Read the model definition and answer for the solid it produces. Units are mm, in the model's axes. Face numbers are marked on the shaded views. A direction names the side the tool comes from. Coordinates: 2 decimals unless noted, no trailing zeros. Write each loop counter-clockwise with the first axis right and the second up, starting at its lowest first coordinate (ties: lowest second). Pieces come first, ordered by that corner, then holes. Notation, with made-up numbers: M 32.5,7 L 74.5,7 A20 ccw 74.5,22 Z; hole C 5,73.5 d7. An arc over 180 degrees is marked long. Write item = value, one per line.
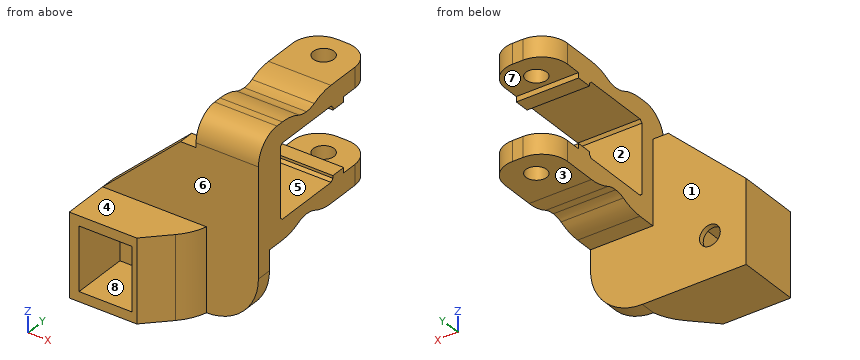
from build123d import *

# Parameters (mm, degrees)
ESQUISSE1_W                   = 30
ESQUISSE1_H                   = 40
BOSS_EXTRU_1_DEPTH            = 3
ESQUISSE8_W                   = 17
ESQUISSE8_H                   = 3.5
BOSS_EXTRU_2_DEPTH            = 20
ESQUISSE11_W                  = 3.5
ESQUISSE11_H                  = 20
ENL_V_MAT_EXTRU_9_DEPTH       = 5
ESQUISSE19_W                  = 12
ESQUISSE19_H                  = 20
BOSS_EXTRU_6_DEPTH            = 16.5
ESQUISSE20_W                  = 14.2
ESQUISSE20_H                  = 14.2
ENL_V_MAT_EXTRU_11_DEPTH      = 50.527769988
ESQUISSE29_W                  = 12
ESQUISSE29_H                  = 3
BOSS_EXTRU_9_DEPTH            = 17
ESQUISSE30_W                  = 12
ESQUISSE30_H                  = 23
BOSS_EXTRU_10_DEPTH           = 1
ESQUISSE31_W                  = 12
ESQUISSE31_H                  = 20
BOSS_EXTRU_11_DEPTH           = 1
ESQUISSE32_W                  = 12.2
ESQUISSE32_H                  = 2.9
ENL_V_MAT_EXTRU_12_DEPTH      = 50.527769988
ESQUISSE33_W                  = 12
ESQUISSE33_H                  = 3.9
BOSS_EXTRU_12_DEPTH           = 8
CONG_6_R                      = 5
ENL_V_MAT_EXTRU_14_DEPTH      = 53.417083332
ENL_V_MAT_EXTRU_14_DEPTH_BACK = 53.417083332
ESQUISSE36_R                  = 2
CHANFREIN1_SIZE               = 0.5
CONG_7_R                      = 5
ENL_V_MAT_EXTRU_15_DEPTH      = 54.712196008
CONG_8_R                      = 10
CONG_9_R                      = 10
ESQUISSE39_W                  = 30
ESQUISSE39_H                  = 3
BOSS_EXTRU_13_DEPTH           = 2
ESQUISSE40_W                  = 18
ESQUISSE40_H                  = 3
BOSS_EXTRU_14_DEPTH           = 2
ESQUISSE38_R                  = 2
ENL_V_MAT_EXTRU_16_DEPTH      = 61.207973065
ESQUISSE41_W                  = 14
ESQUISSE41_H                  = 16
ESQUISSE41_W_2                = 10
ESQUISSE41_H_2                = 12
BOSS_EXTRU_15_DEPTH           = 9
ESQUISSE42_W                  = 10
ESQUISSE42_H                  = 12
ENL_V_MAT_EXTRU_17_DEPTH      = 2
ESQUISSE43_W                  = 30
ESQUISSE43_H                  = 14
ENL_V_MAT_EXTRU_19_DEPTH      = 3
CONG_10_R                     = 10
ESQUISSE44_W                  = 6
ESQUISSE44_H                  = 16
BOSS_EXTRU_16_DEPTH           = 9
CHANFREIN2_SIZE               = 7
CONG_11_R                     = 10
ESQUISSE46_W                  = 10.2
ESQUISSE46_H                  = 12.2
ENL_V_MAT_EXTRU_20_DEPTH      = 11


with BuildPart() as part:
    # Esquisse1 → Boss.-Extru.1 (new body)
    with BuildSketch(Plane(origin=(0, 0, 0), x_dir=(1, 0, 0), z_dir=(0, 1, 0))):
        with Locations((15, 20)):
            Rectangle(ESQUISSE1_W, ESQUISSE1_H)
    extrude(amount=BOSS_EXTRU_1_DEPTH)

    # Esquisse8 → Boss.-Extru.2 (add)
    with BuildSketch(Plane(origin=(0, 3, 0), x_dir=(1, 0, 0), z_dir=(0, 1, 0))):
        with Locations((21.5, 11.375)):
            Rectangle(ESQUISSE8_W, ESQUISSE8_H)
    extrude(amount=BOSS_EXTRU_2_DEPTH)

    # Esquisse11 → Enlèv. mat.-Extru.9 (cut)
    with BuildSketch(Plane.ZY.offset(-13)):
        with Locations((-11.375, 13)):
            Rectangle(ESQUISSE11_W, ESQUISSE11_H)
    extrude(amount=-ENL_V_MAT_EXTRU_9_DEPTH, mode=Mode.SUBTRACT)

    # Esquisse19 → Boss.-Extru.6 (add)
    with BuildSketch(Plane.XY.offset(-9.625)):
        with Locations((24, 13)):
            Rectangle(ESQUISSE19_W, ESQUISSE19_H)
    extrude(amount=BOSS_EXTRU_6_DEPTH)

    # Esquisse20 → Enlèv. mat.-Extru.11 (cut, through all)
    with BuildSketch(Plane.ZY.offset(-18)):
        with Locations((-3.125, 13)):
            Rectangle(ESQUISSE20_W, ESQUISSE20_H)
    extrude(amount=-ENL_V_MAT_EXTRU_11_DEPTH, mode=Mode.SUBTRACT)

    # Esquisse29 → Boss.-Extru.9 (add)
    with BuildSketch(Plane.XY.offset(6.875)):
        with Locations((24, 1.5)):
            Rectangle(ESQUISSE29_W, ESQUISSE29_H)
    extrude(amount=-BOSS_EXTRU_9_DEPTH)

    # Esquisse30 → Boss.-Extru.10 (add)
    with BuildSketch(Plane.XY.offset(6.875)):
        with Locations((24, 11.5)):
            Rectangle(ESQUISSE30_W, ESQUISSE30_H)
    extrude(amount=BOSS_EXTRU_10_DEPTH)

    # Esquisse31 → Boss.-Extru.11 (add)
    with BuildSketch(Plane(origin=(0, 0, -13.125), x_dir=(-1, 0, 0), z_dir=(0, 0, -1))):
        with Locations((-24, 13)):
            Rectangle(ESQUISSE31_W, ESQUISSE31_H)
    extrude(amount=BOSS_EXTRU_11_DEPTH)

    # Esquisse32 → Enlèv. mat.-Extru.12 (cut, through all)
    with BuildSketch(Plane.ZY.offset(-18)):
        with Locations((-3.125, 21.55)):
            Rectangle(ESQUISSE32_W, ESQUISSE32_H)
    extrude(amount=-ENL_V_MAT_EXTRU_12_DEPTH, mode=Mode.SUBTRACT)

    # Esquisse33 → Boss.-Extru.12 (add)
    with BuildSketch(Plane(origin=(0, 23, 0), x_dir=(1, 0, 0), z_dir=(0, 1, 0))):
        with Locations((24, 12.175)):
            Rectangle(ESQUISSE33_W, ESQUISSE33_H)
        with Locations((24, -5.925)):
            Rectangle(ESQUISSE33_W, ESQUISSE33_H)
    extrude(amount=BOSS_EXTRU_12_DEPTH)

    # Congé6
    cong_6_edges = [part.edges().sort_by_distance(p)[0] for p in [
        (18, 31, -12.175),
        (30, 31, -12.175),
        (18, 31, 5.925),
        (30, 31, 5.925),
    ]]
    fillet(cong_6_edges, radius=CONG_6_R)

    # Esquisse36 → Enlèv. mat.-Extru.14 (cut, two sides: drawn at the far end of the back side and taken through both)
    with BuildSketch(Plane.XY.offset(-10.225).offset(-ENL_V_MAT_EXTRU_14_DEPTH_BACK)):
        with Locations((24, 26)):
            Circle(ESQUISSE36_R)
    extrude(amount=ENL_V_MAT_EXTRU_14_DEPTH + ENL_V_MAT_EXTRU_14_DEPTH_BACK, mode=Mode.SUBTRACT)

    # Chanfrein1
    chanfrein1_edges = [part.edges().sort_by_distance(p)[0] for p in [
        (24, 5.9, -10.225),
        (24, 20.1, -10.225),
        (24, 20.1, 3.975),
        (24, 5.9, 3.975),
    ]]
    chamfer(chanfrein1_edges, length=CHANFREIN1_SIZE)

    # Congé7
    cong_7_edges = [part.edges().sort_by_distance(p)[0] for p in [
        (24, 0, 7.875),
    ]]
    fillet(cong_7_edges, radius=CONG_7_R)

    # Esquisse37 → Enlèv. mat.-Extru.15 (cut, through all)
    with BuildSketch(Plane.ZY.offset(-18)):
        with BuildLine():
            Line((-14.125, 16), (-14.125, 10))
            add(Edge.make_bspline(
                [(-14.125, 10), (-12.780635922, 10.344634173), (-12.625, 13)],
                knots=[0, 0, 0, 1, 1, 1], degree=2))
            add(Edge.make_bspline(
                [(-14.125, 16), (-12.780635922, 15.655365827), (-12.625, 13)],
                knots=[0, 0, 0, 1, 1, 1], degree=2))
        make_face()
        with BuildLine():
            Line((7.875, 16), (7.875, 10))
            add(Edge.make_bspline(
                [(7.875, 10), (6.530635922, 10.344634173), (6.375, 13)],
                knots=[0, 0, 0, 1, 1, 1], degree=2))
            add(Edge.make_bspline(
                [(7.875, 16), (6.530635922, 15.655365827), (6.375, 13)],
                knots=[0, 0, 0, 1, 1, 1], degree=2))
        make_face()
    extrude(amount=-ENL_V_MAT_EXTRU_15_DEPTH, mode=Mode.SUBTRACT)

    # Congé8
    cong_8_edges = [part.edges().sort_by_distance(p)[0] for p in [
        (24, 10, 7.875),
        (24, 16, 7.875),
    ]]
    fillet(cong_8_edges, radius=CONG_8_R)

    # Congé9
    cong_9_edges = [part.edges().sort_by_distance(p)[0] for p in [
        (24, 16, -14.125),
        (24, 10, -14.125),
    ]]
    fillet(cong_9_edges, radius=CONG_9_R)

    # Esquisse39 → Boss.-Extru.13 (add)
    with BuildSketch(Plane(origin=(0, 0, -40), x_dir=(-1, 0, 0), z_dir=(0, 0, -1))):
        with Locations((-15, 1.5)):
            Rectangle(ESQUISSE39_W, ESQUISSE39_H)
    extrude(amount=BOSS_EXTRU_13_DEPTH)

    # Esquisse40 → Boss.-Extru.14 (add)
    with BuildSketch(Plane.XY):
        with Locations((9, 1.5)):
            Rectangle(ESQUISSE40_W, ESQUISSE40_H)
    extrude(amount=BOSS_EXTRU_14_DEPTH)

    # Esquisse38 → Enlèv. mat.-Extru.16 (cut, through all)
    with BuildSketch(Plane.XZ):
        with Locations(Location((7, -20, 0), (0, 0, 270))):
            Circle(ESQUISSE38_R)
    extrude(amount=-ENL_V_MAT_EXTRU_16_DEPTH, mode=Mode.SUBTRACT)

    # Esquisse41 → Boss.-Extru.15 (add)
    with BuildSketch(Plane.XZ):
        with Locations((7, -20)):
            Rectangle(ESQUISSE41_W, ESQUISSE41_H)
        with Locations((7, -20)):
            Rectangle(ESQUISSE41_W_2, ESQUISSE41_H_2, mode=Mode.SUBTRACT)
    extrude(amount=BOSS_EXTRU_15_DEPTH)

    # Esquisse42 → Enlèv. mat.-Extru.17 (cut)
    with BuildSketch(Plane.XZ):
        with Locations((7, -20)):
            Rectangle(ESQUISSE42_W, ESQUISSE42_H)
    extrude(amount=-ENL_V_MAT_EXTRU_17_DEPTH, mode=Mode.SUBTRACT)

    # Esquisse43 → Enlèv. mat.-Extru.19 (cut)
    with BuildSketch(Plane.XZ):
        with Locations((15, -35)):
            Rectangle(ESQUISSE43_W, ESQUISSE43_H)
        Polygon((0, -12), (0, 2), (15, 2), align=None)
    extrude(amount=-ENL_V_MAT_EXTRU_19_DEPTH, mode=Mode.SUBTRACT)

    # Congé10
    cong_10_edges = [part.edges().sort_by_distance(p)[0] for p in [
        (30, 1.5, -28),
    ]]
    fillet(cong_10_edges, radius=CONG_10_R)

    # Esquisse44 → Boss.-Extru.16 (add)
    with BuildSketch(Plane.XZ):
        with Locations((17, -20)):
            Rectangle(ESQUISSE44_W, ESQUISSE44_H)
    extrude(amount=BOSS_EXTRU_16_DEPTH)

    # Chanfrein2
    chanfrein2_edges = [part.edges().sort_by_distance(p)[0] for p in [
        (20, -9, -20),
    ]]
    chamfer(chanfrein2_edges, length=CHANFREIN2_SIZE)

    # Congé11
    # the kernel refuses this fillet: 10 mm, written as the material it takes off along each edge
    with BuildSketch(Plane(origin=(20, -2, -2.718486848), x_dir=(-0.7071067811865474, -0.7071067811865477, 0), z_dir=(0, 0, -1))) as cong_11_piece_1:
        with BuildLine():
            CenterArc((3.712605261, 10), CONG_11_R, 239.157365729, 30.842634271)
            Line((-1.414213562, 1.414213562), (-1.516749939, 1.242497834))
            ThreePointArc((-1.516749939, 1.242497834), (-0.848528137, 0.565685425), (-0.141421356, -0.141421356))
            Line((-0.141421356, -0.141421356), (0, -0.2))
            Line((0, -0.2), (3.712605261, -0.2))
            Line((3.712605261, -0.2), (3.712605261, 0))
        make_face()
    extrude(amount=34.563026305, mode=Mode.SUBTRACT)

    # Esquisse46 → Enlèv. mat.-Extru.20 (cut)
    with BuildSketch(Plane.XZ.offset(9)):
        with Locations((7, -20)):
            Rectangle(ESQUISSE46_W, ESQUISSE46_H)
    extrude(amount=-ENL_V_MAT_EXTRU_20_DEPTH, mode=Mode.SUBTRACT)


solid = part.part
Item 1: Find section B-B (z = -20). Determine the outline of the cut face in (x, y).
Worked answers:
outline = M 0,-9 L 1.9,-9 L 1.9,2 L 5,2 L 5,3 L 0,3 Z; M 9,2 L 12.1,2 L 12.1,-9 L 13,-9 L 17.37,-4.63 A10 ccw 20,0 L 29.8,0 L 29.8,3 L 9,3 Z
Item 2: Which of the six approach directions +Z, -Z, +X, -X, +Y, -Y give full straight-line access (tool end or side, diameter ignored) to the marked faces 4, 5, 6, 7 and 8?
Worked answers:
face_4 = +Z, +X, -X, -Y
face_5 = +X, -X
face_6 = +Z, +X, -Y
face_7 = +X, -X, +Y
face_8 = -Y
Item 3: For a pull along Z with two mould halves and no side action, classify the marked faces 1, 2 and 3 as released by +Z, released by -Z, zero draft, split by the parting line, or undercut.
Worked answers:
face_1 = zero draft
face_2 = undercut
face_3 = released by -Z
Item 4: Find section D-D (z = -24). Determine the outline of the cut face in (x, y), and give its area (3 significant figures).
Worked answers:
outline = M 0,-9 L 1.9,-9 L 1.9,2 L 12.1,2 L 12.1,-9 L 13,-9 L 17.37,-4.63 A10 ccw 20,0 L 28,0 L 28,3 L 0,3 Z
area = 126 mm²
Item 5: Consider line 1 along X through (y, z) = (26, -12); line 2 along Y through (x, z) = (24, -13.3); line 3 along Y through (x, z) = (24, -12). Determine where each line is inside the solid, lowest interval first. Write a range as from..to.
Worked answers:
line_1 = 18..22, 26..30
line_2 = 0..10.44, 15.56..24, 28..31
line_3 = 0..24, 28..31
Item 6: Find section A-A (y = 22). Determine the outline of the cut face in (x, z) (3 decimals), and give its area (3 significant figures).
Worked answers:
outline = M 18,-14.125 L 30,-14.125 L 30,-9.225 L 18,-9.225 Z; M 18,2.975 L 30,2.975 L 30,7.875 L 18,7.875 Z
area = 118 mm²
Item 7: Flat-ended cylindrical pins translate along their axes: pin 1 (3 mm diameter, centred on x = 24, y = 26, fed in from +Z); pin 2 (0.9 mm diameter, centred on x = 23.5, y = 21.5, fed in from -Z) (3 decimals); pin 3 (8 mm diameter, centred on y = 13.5, z = -13.5, fed in from +X); pin 4 (6 mm diameter, centred on x = 23.5, y = 10.5, fed in from +Z). Find the tip coordinate at first contact, or state that the pin passes through.
Worked answers:
pin_1 = through
pin_2 = -14.125
pin_3 = 30
pin_4 = 7.82
Item 8: Find section C-C (x = 6.5). Determine the outline of the cut face in (y, z).
Worked answers:
outline = M -9,-28 L 3,-28 L 3,-21.94 L 2,-21.94 L 2,-26.1 L -9,-26.1 Z; M -9,-13.9 L 2,-13.9 L 2,-18.06 L 3,-18.06 L 3,-5.93 L 0,-5.93 L 0,-12 L -9,-12 Z
